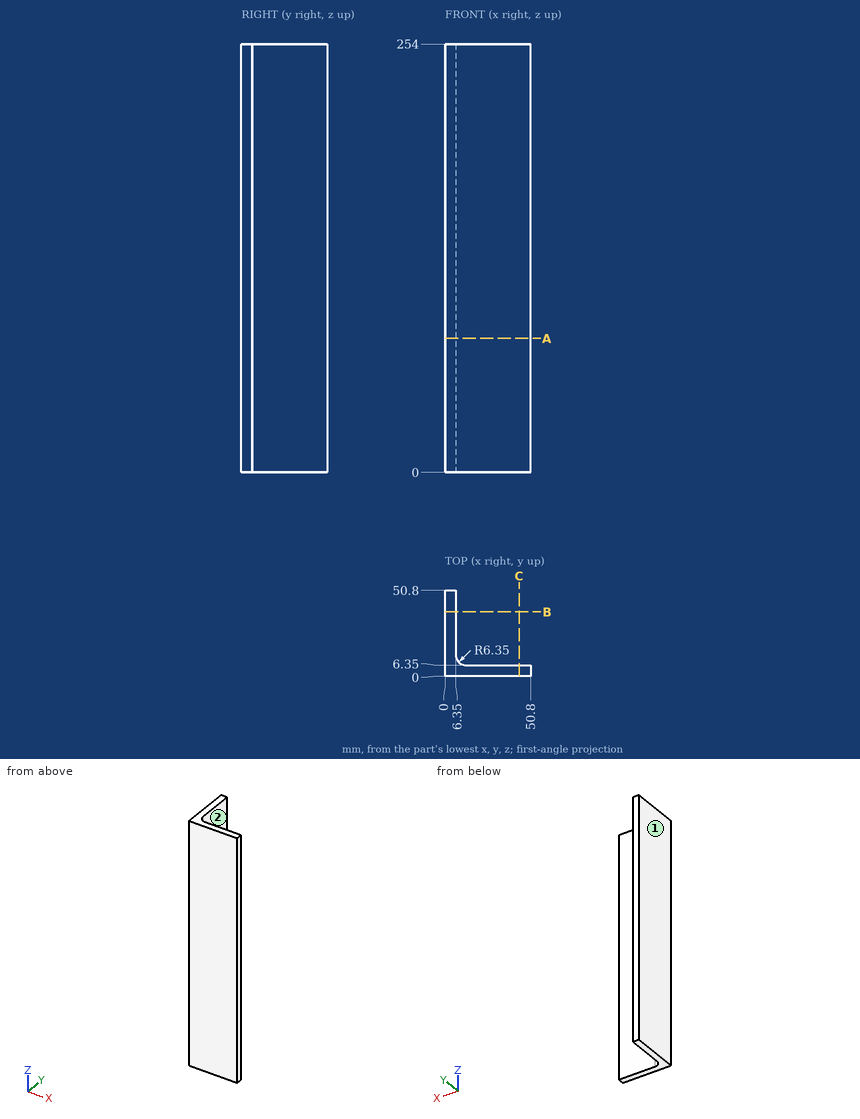
The drawing under review shows one solid part. Ordinate dimensions are in mm from its lowest x, y, z. A direction names the side the tool comes from. Round coordinates to 2 decimals unless told otherwise and drop trailing zeros. Write each loop counter-clockwise with the first axis right and the second up, starting at its lowest first coordinate (ties: lowest second). Pieces come first, ordered by that corner, then holes. Notation, with made-up numbers: (72, -25.5) - (86, -25.5) arc R22 cw to (86, 12.5) - close; hole circle Ø8 at (72.25, -9.75). An arc over 180 degrees is marked (long way). Use a Markdown table: item, result. Add a question column.
1. We need section B-B (y = 38). State the section outline as (x, z) points.
2. Wall thickness on probe 1 along Y at (x, z) = (21.5, 164); probe 2 along X at (y, z) = (8, 102): over which ranges is each line inside the solid? List them lowest first.
3. For the marked faces 1 and 2, list the 3-axis set-ups (+Z, -Z, +X, -X, +Y, -Y) from which the entire face can be reached by the end or side of a thin tool; tool diameter is ignored.
4. We need section A-A (z = 79.5). State the section outline as (x, y) points, then the cut area to 3 significant figures.
5. Clearance check with flat-ended pins moving along their axes: pin 1 (4 mm diameter, centred on x = 20.5, z = 64.5, fed in from +Y); pin 2 (4 mm diameter, centred on x = 17.5, y = 9.5, fed in from +Z); pin 3 (3 mm diameter, centred on y = 24, z = 216.5, fed in from +X). State where each tip first meets the part, or that it passes through.
Output:
| question | item | result |
|---|---|---|
| 1 | outline | (0, 0) - (6.35, 0) - (6.35, 254) - (0, 254) - close |
| 2 | probe 1 | y = 0 to 6.35 |
| 2 | probe 2 | x = 0 to 8.43 |
| 3 | face 1 | +Z, -Z, -X, +Y, -Y |
| 3 | face 2 | +Z, -Z, +X, +Y |
| 4 | outline | (0, 0) - (50.8, 0) - (50.8, 6.35) - (12.7, 6.35) arc R6.35 cw to (6.35, 12.7) - (6.35, 50.8) - (0, 50.8) - close |
| 4 | area | 613 mm2 |
| 5 | pin 1 | stops at y = 6.35 |
| 5 | pin 2 | passes through |
| 5 | pin 3 | stops at x = 6.35 |
